from build123d import *

# Parameters (mm, degrees)
SKETCH1_R                = 29.0703
BOSS_EXTRUDE2_DEPTH      = 4.7625
FILLET1_R                = 3.175
SKETCH2_W                = 14.732
SKETCH2_H                = 10.414
CUT_EXTRUDE2_DEPTH       = 12.7
CIRPATTERN1_COUNT        = 7
SKETCH4_R                = 1.143
CUT_EXTRUDE4_DEPTH       = 9.525
CIRPATTERN2_COUNT        = 7
SKETCH6_R                = 1.905
CUT_EXTRUDE7_DEPTH       = 42.376236281
BOSS_EXTRUDE4_REACH      = 48.843
FILLET2_R                = 0.127
CIRPATTERN5_COUNT        = 7
FILLET2_OF_CIRPATTERN5_R = 0.127
CUT_EXTRUDE9_REACH       = 43.376
SKETCH5_R                = 4.7625


with BuildPart() as part:
    # Sketch1 → Boss-Extrude2 (new body)
    with BuildSketch(Plane.XY):
        Circle(SKETCH1_R)
    extrude(amount=-BOSS_EXTRUDE2_DEPTH)

    # Fillet1
    fillet1_edges = [part.edges().sort_by_distance(p)[0] for p in [
        (-29.0703, 0, -4.7625),
    ]]
    fillet(fillet1_edges, radius=FILLET1_R)

    # Sketch2 → Cut-Extrude2 (cut)
    with BuildSketch(Plane.XY):
        with Locations((0, 25.1333)):
            Rectangle(SKETCH2_W, SKETCH2_H)
    cut_extrude2 = extrude(amount=-CUT_EXTRUDE2_DEPTH, mode=Mode.SUBTRACT)

    # CirPattern1: Cut-Extrude2 ×7 about axis
    cirpattern1_axis = Axis((0, 0, 0), (0, 0, 1))
    for i in range(1, CIRPATTERN1_COUNT):
        add(cut_extrude2.rotate(cirpattern1_axis, i * 360 / CIRPATTERN1_COUNT), mode=Mode.SUBTRACT)

    # Sketch4 → Cut-Extrude4 (cut, symmetric)
    with BuildSketch(Plane(origin=(0, 0, 0), x_dir=(0, 0, -1), z_dir=(1, 0, 0))):
        with Locations((0, 25.7683)):
            Circle(SKETCH4_R)
    cut_extrude4 = extrude(amount=CUT_EXTRUDE4_DEPTH, both=True, mode=Mode.SUBTRACT)

    # CirPattern2: Cut-Extrude4 ×7 about axis
    cirpattern2_axis = Axis((0, 0, 0), (0, 0, 1))
    for i in range(1, CIRPATTERN2_COUNT):
        add(cut_extrude4.rotate(cirpattern2_axis, i * 360 / CIRPATTERN2_COUNT), mode=Mode.SUBTRACT)

    # Sketch6 → Cut-Extrude7 (cut, through all)
    with BuildSketch(Plane(origin=(0, 0, -4.7625), x_dir=(-1, 0, 0), z_dir=(0, 0, -1))):
        with Locations((0, -12.7)):
            Circle(SKETCH6_R)
        with Locations((-10.998522628, 6.35)):
            Circle(SKETCH6_R)
        with Locations((10.998522628, 6.35)):
            Circle(SKETCH6_R)
    extrude(amount=-CUT_EXTRUDE7_DEPTH, mode=Mode.SUBTRACT)

    # Sketch10 → Boss-Extrude4 (add, up to next)
    with BuildSketch(Plane.ZY.offset(-7.366), mode=Mode.PRIVATE) as boss_extrude4_sk1:
        with BuildLine():
            Line((-4.7625, 19.9263), (0, 19.9263))
            Line((0, 19.9263), (0, 20.0533))
            ThreePointArc((0, 20.0533), (-2.7025038, 20.73265722), (-4.7625, 22.609214887))
            Line((-4.7625, 22.609214887), (-4.7625, 19.9263))
        make_face()
    boss_extrude4_tool1 = extrude(boss_extrude4_sk1.sketch, amount=BOSS_EXTRUDE4_REACH, mode=Mode.PRIVATE) - part.part
    boss_extrude4 = boss_extrude4_tool1.solids().sort_by_distance((7.366, 20.664807, -3.452063))[0]
    add(boss_extrude4)

    # Fillet2
    fillet2_edges = [part.edges().sort_by_distance(p)[0] for p in [
        (0, 22.609214887, -4.7625),
    ]]
    fillet(fillet2_edges, radius=FILLET2_R)

    # CirPattern5: Boss-Extrude4 ×7 about axis
    cirpattern5_axis = Axis((0, 0, 0), (0, 0, 1))
    for i in range(1, CIRPATTERN5_COUNT):
        add(boss_extrude4.rotate(cirpattern5_axis, i * 360 / CIRPATTERN5_COUNT))

    # Fillet2 of CirPattern5
    fillet2_of_cirpattern5_edges = [part.edges().sort_by_distance(p)[0] for p in [
        (-17.676595993, 14.09661491, -4.7625),
        (-22.042354666, -5.031023613, -4.7625),
        (-9.809770694, -20.370198741, -4.7625),
        (9.809770694, -20.370198741, -4.7625),
        (22.042354666, -5.031023613, -4.7625),
        (17.676595993, 14.09661491, -4.7625),
    ]]
    fillet(fillet2_of_cirpattern5_edges, radius=FILLET2_OF_CIRPATTERN5_R)

    # Sketch5 → Cut-Extrude9 (cut, up to next)
    with BuildSketch(Plane.XY, mode=Mode.PRIVATE) as cut_extrude9_sk1:
        Circle(SKETCH5_R)
    cut_extrude9_tool1 = extrude(cut_extrude9_sk1.sketch, amount=-CUT_EXTRUDE9_REACH, mode=Mode.PRIVATE) & part.part
    add(cut_extrude9_tool1.solids().sort_by_distance((0, 0, 0))[0], mode=Mode.SUBTRACT)


solid = part.part
Source: CAD feature listing. Evaluate the final solid. Frame: model axes, mm. A direction names the side the tool comes from. Give positions to 0.01 mm unless a question says otherwise; leave off trailing zeros. Write item = value, one per line.
Q1. Pull-direction query (Y, two-part tool) for faces 1 (the face through (23.215, -13.977, -1.143)), 2 (the face through (23.381, 9.224, -2.348)), 3 (the face through (-17.063, -18.455, -2.348)); classes: released by +Y, released by -Y, zero draft, split by the parting line, or undercut.
Data:
face_1 = undercut
face_2 = released by +Y
face_3 = released by -Y
Q2. Pin query (flat end, axial travel): pin 1 (1 mm diameter, centred on y = -21.5, z = -3, fed in from -X); pin 2 (1.3 mm diameter, centred on y = 25.5, z = -0.5, fed in from +X); pin 3 (1.4 mm diameter, centred on y = 26, z = -1.5, fed in from -X). Return the tip coordinate at first contact, or that it passes through.
Data:
pin_1 = -19.71
pin_2 = 15.09
pin_3 = -14.32
Q3. Cut plane A-A, the plane z = -2.55. State how many separate pieces and enclosed holes the cut face has, and give its area (3 significant figures).
Data:
separate_pieces = 1
enclosed_holes = 4
area = 1,700 mm^2
Q4. Set-up query: faces 4 (the face through (-7.366, 24, -2)), 5 (the face through (-21.79, -12.53, -2.35)), 6 (the face through (8.461, 25.743, -1.143)), 7 (the face through (14.196, 20.742, -2.348)). Return all of +Z, -Z, +X, -X, +Y, -Y with unobstructed straight access to the full face (end or side cutting, diameter ignored); none if empty.
Data:
face_4 = +Z, +Y
face_5 = +Z, -X
face_6 = +Z
face_7 = +Z, +X
Q5. Material intervals for line 1 (Y direction, x = 0, z = -1.35) (1 decimal); line 2 (X direction, y = -16.5, z = -2.4); line 3 (Y direction, x = 0, z = -2.35) (1 decimal), sorted ascending. Write a range as from..to.
Data:
line_1 = -29.1..-14.6, -10.8..-4.8, 4.8..20.2
line_2 = -23.81..-16.12, -13.17..13.17, 16.12..23.81
line_3 = -29..-14.6, -10.8..-4.8, 4.8..20.6
